```python
from build123d import *

# Parameters (mm, degrees)
F0_R     = 26
F1_DEPTH = 3
F2_R     = 26
F2_R_2   = 23.75
F3_DEPTH = 70
F5_D     = 5


with BuildPart() as f1:
    # F0 (on Front) → F1 (new body)
    with BuildSketch(Plane.XZ):
        Circle(F0_R)
    extrude(amount=F1_DEPTH)

    # F2 (on face) → F3 (join)
    with BuildSketch(Plane.XZ.offset(3)):
        Circle(F2_R)
        Circle(F2_R_2, mode=Mode.SUBTRACT)
    extrude(amount=F3_DEPTH)

    # F5 (through all)
    with Locations(Plane(origin=(0, 0, 0), x_dir=(-1, 0, 0), z_dir=(0, 1, 0))):
        with Locations((0, 0)):
            Hole(F5_D / 2)


solid = f1.part
```
Work out the finished part from the listing and answer in its coordinate system (mm). A direction names the side the tool comes from. Coordinates: 2 decimals unless noted, no trailing zeros. Loops run counter-clockwise (first coordinate to the right, second up) from the corner with the lowest first, then second, coordinate; pieces in that order, holes last. Notation, with made-up numbers: M 45,-34 L 70,-34 A17 ccw 70,-3 Z; hole C 78,29.5 d7. An arc over 180 degrees is marked long. Use CSV: the item, a comma, the result in double quotes. Start each with the question number.
(1) Find section A-A, the plane x = 0. Give the vertices of the cut face in (y, z).
(2) Consider line 1 (Z direction, x = 0, y = -1.6); line 2 (Y direction, x = -5, z = -10.5); line 3 (X direction, y = -59, z = -1). Determine where each line is inside the solid, lowest interval first.
(3) Find section D-D, the plane y = -43.5. Give the vertices of the cut face in (x, z).
(4) Find section C-C, the plane x = -9. Give the vertices of the cut face in (y, z).
(5) Given pin 1 Ø3 at (x, y) = (3.5, -34.5) entering from -Z; pin 2 Ø1 at (x, z) = (-4, 20) entering from -Y; pin 3 Ø1.5 at (x, y) = (0, -21.5) entering from +Z, each flat-ended and moving along its own axis, determine where each tip first touches the part or whether it passes through.
(6) Find section B-B, the plane z = 0. Give the vertices of the cut face in (x, y).
(7) For a pull along X with two mould halves and no side action, classify faces 1 (the face through (-5.149, -37.51, -23.185)), 2 (the face through (5, 0, 0)), 3 (the face through (-20.633, -35.989, -15.821)) as +X half, -X half, draft (parallel to the pull), parting line (faces both ways), or undercut.
(8) For faces 4 (the face through (5, -3, 0)), 5 (the face through (11.4, -73, -21.1)), determine the directions among +Z, -Z, +X, -X, +Y, -Y from which every point of the face is accessible in a straight line to the end or side of a thin tool.
Recorded:
1,outline,"M -73,-26 L 0,-26 L 0,-2.5 L -3,-2.5 L -3,-23.75 L -73,-23.75 Z; M -73,23.75 L -3,23.75 L -3,2.5 L 0,2.5 L 0,26 L -73,26 Z"
2,line 1,"z = -26 to -2.5, 2.5 to 26"
2,line 2,"y = -3 to 0"
2,line 3,"x = -25.98 to -23.73, 23.73 to 25.98"
3,outline,"C 0,0 d52; hole C 0,0 d47.5"
4,outline,"M -73,-24.39 L 0,-24.39 L 0,24.39 L -73,24.39 L -73,21.98 L -3,21.98 L -3,-21.98 L -73,-21.98 Z"
5,pin 1,"stops at z = -25.92"
5,pin 2,"stops at y = -3"
5,pin 3,"stops at z = 26"
6,outline,"M -26,-73 L -23.75,-73 L -23.75,-3 L -2.5,-3 L -2.5,0 L -26,0 Z; M 2.5,-3 L 23.75,-3 L 23.75,-73 L 26,-73 L 26,0 L 2.5,0 Z"
7,face 1,"undercut"
7,face 2,"draft"
7,face 3,"parting line"
8,face 4,"-Y"
8,face 5,"+Z, -Z, +X, -X, -Y"
